The model under review builds one solid part; all positions refer to its coordinate system, in mm. Coordinates: 2 decimals unless noted, no trailing zeros. Loops run counter-clockwise (first coordinate to the right, second up) from the corner with the lowest first, then second, coordinate; pieces in that order, holes last. Notation, with made-up numbers: (-9, 35) - (39, 35) arc R29 ccw to (39, 74) - close; hole circle Ø10 at (-12.5, 50). An arc over 180 degrees is marked (long way). Answer in a Markdown table with one row per item. Add a question column.
(1) For P1, Ø2, axis at x = -4, z = -2.5, coming from the +Y side; P2, Ø1.6, axis at y = 0.5, z = 14.5, coming from the +X side; P3, Ø1, axis at y = 1, z = 17, coming from the -X side; P4, Ø1.2, axis at x = 2.5, z = -0.5, coming from the +Y side, all flat-tipped, find the tip position at first contact; note any pin that passes through.
(2) We need section D-D on x = 8.5. Write out the cut boundary in (y, z), plus the area to 3 significant figures.
(3) We need section B-B on z = 0. Write out the cut boundary in (x, y).
(4) We need section C-C on z = 6. Write out the cut boundary in (x, y).
(5) For line 1 along X through (y, z) = (0.7, 0); line 2 along Z through (x, y) = (0.25, 1.85); line 3 along X through (y, z) = (0.95, -2.5), list the stretches that pass through material, from the lowest coordinate up.
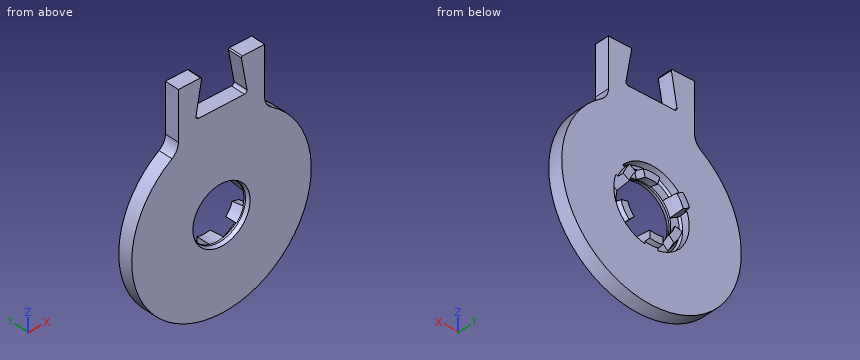
from build123d import *

# Parameters (mm, degrees)
SKETCH1_R                = 4
BOSS_EXTRUDE1_DEPTH      = 2
SKETCH2_R                = 12.5
SKETCH2_R_2              = 3.8
BOSS_EXTRUDE2_DEPTH      = 2
SKETCH4_W                = 12
SKETCH4_H                = 0.2
CUT_EXTRUDE1_DEPTH       = 4
FILLET3_R                = 0.35
FILLET4_R                = 0.15
FILLET6_R                = 2
SKETCH13_R               = 5.25
CUT_EXTRUDE5_DEPTH       = 1.25
REVOLVE2_ANGLE           = 30
CIRPATTERN2_COUNT        = 3
CHAMFER1_SIZE            = 0.5
CHAMFER1_SIZE2           = 0.181985117
FILLET14_R               = 0.25
BOSS_EXTRUDE8_DEPTH      = 2
BOSS_EXTRUDE8_DRAFT      = -3
SKETCH16_W               = 2
SKETCH16_H               = 1.934959958
BOSS_EXTRUDE9_DEPTH      = 1.25
BOSS_EXTRUDE9_TAPER      = 3
CIRPATTERN3_COUNT        = 3
CIRPATTERN3_COPY_1_DEPTH = 2
CIRPATTERN3_COPY_1_DRAFT = -3
CIRPATTERN3_COPY_2_DEPTH = 2
CIRPATTERN3_COPY_2_DRAFT = -3


with BuildPart() as part:
    # Sketch1 → Boss-Extrude1 (new body)
    with BuildSketch(Plane(origin=(0, 0, 0), x_dir=(1, 0, 0), z_dir=(0, 1, 0))):
        Polygon((-6, 6), (-6, -13.291502622), (-6, -19), (-2.70227506, -19), (-3.619175359, -13.8), (0, -13.8), (3.619175359, -13.8), (2.70227506, -19), (6, -19), (6, -13.291502622), (6, 6), align=None)
        with Locations(Location((0, 0, 0), (0, 0, 270))):
            Circle(SKETCH1_R, mode=Mode.SUBTRACT)
    extrude(amount=BOSS_EXTRUDE1_DEPTH)

    # Sketch2 → Boss-Extrude2 (add)
    with BuildSketch(Plane(origin=(0, 0, 0), x_dir=(1, 0, 0), z_dir=(0, 1, 0))):
        Circle(SKETCH2_R)
        with Locations(Location((0, 0, 0), (0, 0, 270))):
            Circle(SKETCH2_R_2, mode=Mode.SUBTRACT)
    extrude(amount=BOSS_EXTRUDE2_DEPTH)

    # Sketch4 → Cut-Extrude1 (cut)
    with BuildSketch(Plane(origin=(0, 2, 0), x_dir=(1, 0, 0), z_dir=(0, 1, 0))):
        with Locations((0, -18.9)):
            Rectangle(SKETCH4_W, SKETCH4_H)
    extrude(amount=-CUT_EXTRUDE1_DEPTH, mode=Mode.SUBTRACT)

    # Fillet3
    fillet3_edges = [part.edges().sort_by_distance(p)[0] for p in [
        (3.619175359, 1, 13.8),
        (-3.619175359, 1, 13.8),
    ]]
    fillet(fillet3_edges, radius=FILLET3_R)

    # Fillet4
    fillet4_edges = [part.edges().sort_by_distance(p)[0] for p in [
        (2.737540456, 1, 18.8),
        (-2.737540456, 1, 18.8),
    ]]
    fillet(fillet4_edges, radius=FILLET4_R)

    # Fillet6
    fillet6_edges = [part.edges().sort_by_distance(p)[0] for p in [
        (6, 1, 10.9658561),
        (-6, 1, 10.9658561),
    ]]
    fillet(fillet6_edges, radius=FILLET6_R)

    # Sketch13 → Cut-Extrude5 (cut)
    with BuildSketch(Plane(origin=(0, 2, 0), x_dir=(1, 0, 0), z_dir=(0, 1, 0))):
        with Locations(Location((0, 0, 0), (0, 0, 270))):
            Circle(SKETCH13_R)
    extrude(amount=-CUT_EXTRUDE5_DEPTH, mode=Mode.SUBTRACT)

    # Sketch12 → Revolve2 (revolve, symmetric)
    with BuildSketch(Plane(origin=(0, 0, 0), x_dir=(0, 0, -1), z_dir=(1, 0, 0))) as revolve2_sk:
        Polygon((-4, 0), (-3.4, 2), (-4.4, 2), (-5, 0), align=None)
    revolve2 = revolve(axis=Axis((0, 0, 0), (0, 1, 0)), revolution_arc=REVOLVE2_ANGLE / 2)
    revolve2 = revolve2 + revolve(revolve2_sk.sketch, axis=Axis((0, 0, 0), (0, -1, 0)), revolution_arc=REVOLVE2_ANGLE / 2)

    # CirPattern2: Revolve2 ×3 about axis
    cirpattern2_axis = Axis((0, 0, 0), (0, 1, 0))
    for i in range(1, CIRPATTERN2_COUNT):
        add(revolve2.rotate(cirpattern2_axis, i * 360 / CIRPATTERN2_COUNT))

    # Chamfer1
    chamfer1_edges = [part.edges().sort_by_distance(p)[0] for p in [
        (0, 0, -3.8),
    ]]
    chamfer1_side = [part.faces().sort_by_distance(p)[0] for p in [
        (0, 0.375, -3.8),
    ]]
    chamfer(chamfer1_edges, length=CHAMFER1_SIZE, length2=CHAMFER1_SIZE2, reference=chamfer1_side[0])

    # Fillet14
    fillet14_edges = [part.edges().sort_by_distance(p)[0] for p in [
        (0, 0.75, -5.25),
        (0, 0.75, 4.775),
        (-4.135271303, 0.75, -2.3875),
        (4.135271303, 0.75, -2.3875),
    ]]
    fillet(fillet14_edges, radius=FILLET14_R)


with BuildPart() as boss_extrude8_tool:
    # Boss-Extrude8: read off the stored shape, not the designer's step
    # Boss-Extrude8 outline → Boss-Extrude8 (with draft: the straight prism first)
    with BuildSketch(Plane.XZ.offset(-2.75)):
        with BuildLine():
            Line((-0.895184441, -3.800819565), (-0.895184441, -4.812637066))
            ThreePointArc((-0.895184441, -4.812637066), (0, -4.895184441), (0.895184441, -4.812637066))
            Line((0.895184441, -4.812637066), (0.895184441, -3.800819565))
            ThreePointArc((0.895184441, -3.800819565), (0, -3.904815559), (-0.895184441, -3.800819565))
        make_face()
    extrude(amount=BOSS_EXTRUDE8_DEPTH)
    # Boss-Extrude8: the draft: its side faces are tilted about the plane it starts from
    boss_extrude8_sides = [boss_extrude8_tool.faces().sort_by_distance(p)[0] for p in [
        (0.895184441, 1.75, -4.306728316),
        (0, 1.75, -3.904815559),
        (-0.895184441, 1.75, -4.306728316),
        (0, 1.75, -4.895184441),
    ]]
    draft(boss_extrude8_sides, Plane.XZ.offset(-2.75), BOSS_EXTRUDE8_DRAFT)


with BuildPart() as part_1:
    add(part.part)

    # Boss-Extrude8: add boss_extrude8_tool
    add(boss_extrude8_tool.part)

    # Sketch16 → Boss-Extrude9 (add)
    with BuildSketch(Plane(origin=(0, 0.75, 0), x_dir=(1, 0, 0), z_dir=(0, 1, 0))):
        with Locations((0, 5.25)):
            Rectangle(SKETCH16_W, SKETCH16_H)
    boss_extrude9 = extrude(amount=BOSS_EXTRUDE9_DEPTH, taper=BOSS_EXTRUDE9_TAPER)

    # CirPattern3: Boss-Extrude9 ×3 about axis
    cirpattern3_axis = Axis((0, 0, 0), (0, 1, 0))
    for i in range(1, CIRPATTERN3_COUNT):
        add(boss_extrude9.rotate(cirpattern3_axis, i * 360 / CIRPATTERN3_COUNT))


with BuildPart() as cirpattern3_copy_1_tool:
    # CirPattern3 copy 1 sketch → CirPattern3 copy 1 (with draft: the straight prism first)
    with BuildSketch(Plane(origin=(0, 2.75, 0), x_dir=(-0.4999999999999998, 0, -0.8660254037844387), z_dir=(0, -1, 0))):
        with BuildLine():
            Line((-0.895184441, -3.800819565), (-0.895184441, -4.812637066))
            ThreePointArc((-0.895184441, -4.812637066), (0, -4.895184441), (0.895184441, -4.812637066))
            Line((0.895184441, -4.812637066), (0.895184441, -3.800819565))
            ThreePointArc((0.895184441, -3.800819565), (0, -3.904815559), (-0.895184441, -3.800819565))
        make_face()
    extrude(amount=CIRPATTERN3_COPY_1_DEPTH)
    # CirPattern3 copy 1: the draft: its side faces are tilted about the plane it starts from
    cirpattern3_copy_1_sides = [cirpattern3_copy_1_tool.faces().sort_by_distance(p)[0] for p in [
        (-4.177328349, 1.75, 1.378111691),
        (-3.381669471, 1.75, 1.952407779),
        (-3.282143908, 1.75, 2.928616625),
        (-4.239354082, 1.75, 2.44759222),
    ]]
    draft(cirpattern3_copy_1_sides, Plane(origin=(0, 2.75, 0), x_dir=(-0.4999999999999998, 0, -0.8660254037844387), z_dir=(0, -1, 0)), CIRPATTERN3_COPY_1_DRAFT)


with BuildPart() as part_2:
    add(part_1.part)

    # CirPattern3 copy 1: add cirpattern3_copy_1_tool
    add(cirpattern3_copy_1_tool.part)


with BuildPart() as cirpattern3_copy_2_tool:
    # CirPattern3 copy 2 sketch → CirPattern3 copy 2 (with draft: the straight prism first)
    with BuildSketch(Plane(origin=(0, 2.75, 0), x_dir=(-0.5000000000000004, 0, 0.8660254037844384), z_dir=(0, -1, 0))):
        with BuildLine():
            Line((-0.895184441, -3.800819565), (-0.895184441, -4.812637066))
            ThreePointArc((-0.895184441, -4.812637066), (0, -4.895184441), (0.895184441, -4.812637066))
            Line((0.895184441, -4.812637066), (0.895184441, -3.800819565))
            ThreePointArc((0.895184441, -3.800819565), (0, -3.904815559), (-0.895184441, -3.800819565))
        make_face()
    extrude(amount=CIRPATTERN3_COPY_2_DEPTH)
    # CirPattern3 copy 2: the draft: its side faces are tilted about the plane it starts from
    cirpattern3_copy_2_sides = [cirpattern3_copy_2_tool.faces().sort_by_distance(p)[0] for p in [
        (3.282143908, 1.75, 2.928616625),
        (3.381669471, 1.75, 1.95240778),
        (4.177328349, 1.75, 1.378111691),
        (4.239354082, 1.75, 2.447592221),
    ]]
    draft(cirpattern3_copy_2_sides, Plane(origin=(0, 2.75, 0), x_dir=(-0.5000000000000004, 0, 0.8660254037844384), z_dir=(0, -1, 0)), CIRPATTERN3_COPY_2_DRAFT)


with BuildPart() as part_3:
    add(part_2.part)

    # CirPattern3 copy 2: add cirpattern3_copy_2_tool
    add(cirpattern3_copy_2_tool.part)


solid = part_3.part
Outcome:
| question | item | result |
|---|---|---|
| 1 | P1 | y = 2 |
| 1 | P2 | x = 6 |
| 1 | P3 | x = -6 |
| 1 | P4 | through |
| 2 | outline | (0, -9.17) - (2, -9.17) - (2, 9.17) - (0, 9.17) - close |
| 2 | area | 36.7 mm² |
| 3 | outline | (-12.5, 0) - (-3.98, 0) - (-3.8, 0.5) - (-3.8, 0.75) - (-5, 0.75) arc R0.25 cw to (-5.25, 1) - (-5.25, 2) - (-12.5, 2) - close; (3.8, 0.5) - (3.98, 0) - (12.5, 0) - (12.5, 2) - (5.25, 2) - (5.25, 1) arc R0.25 cw to (5, 0.75) - (3.8, 0.75) - close |
| 4 | outline | (-10.97, 0) - (10.97, 0) - (10.97, 2) - (-10.97, 2) - close |
| 5 | line 1 | -12.5 to -3.8, 3.8 to 12.5 |
| 5 | line 2 | -12.5 to -3.85, 3.44 to 4.44, 5.24 to 13.8 |
| 5 | line 3 | -12.25 to -4.61, -4 to -2.75, 2.75 to 4, 4.61 to 12.25 |
